Model file for the job. Use its own axes, mm. Face numbers are marked on the shaded views. A direction names the side the tool comes from. Round coordinates to 2 decimals unless told otherwise and drop trailing zeros. Order: outer loops, then holes, each group sorted by start corner. A loop starts at its lowest first (then second) coordinate and runs counter-clockwise, first axis right, second up. Notation, with made-up numbers: M -30,-32 L 15,-32 A23 cw 15,-12 Z; hole C 54.25,-31 d4. An arc over 180 degrees is marked long. Return JSON: item names as keys, results as strings. Group by question number.
Item 1: Pin check, flat tips, straight feed: pin 1 Ø13 at (x, z) = (8, -2.5) entering from -Y; pin 2 Ø5 at (x, z) = (-2, -0.5) entering from +Y. Stop position of each tip, or through.
Item 2: Probe line 1 along Z through (x, y) = (0, -2); line 2 along Z through (x, y) = (-1.5, -6.5); line 3 along X through (y, z) = (-6.25, 5.75). List the from-to ranges inside material, lowest first.
Item 3: Pull direction X, two halves, no side cores. Call the marked faces 3, 4 and 5: pulls with the +X half, pulls with the -X half, needs draft (parallel to the pull), parting line crosses it, or undercut.
Item 4: Slice it at A-A on z = 0. Write the cut outline in (x, y), then the cut area to 3 significant figures.
Item 5: Which spindle directions (+Z, -Z, +X, -X, +Y, -Y) get a long thin tool onto all of the face, cutting with end or side? Do the marked faces 1 and 2. Say none if no direction does.
Item 6: Slice it at B-B on x = -14.5. Write the cut outline in (y, z), then the cut area to 3 significant figures.
Item 7: Slice it at D-D on z = -9.75. Write the cut outline in (x, y).
Item 8: Slice it at C-C on y = -1.5. Write the cut outline in (x, z), then the cut area to 3 significant figures.
from build123d import *

# Parameters (mm, degrees)
F0_W     = 50
F0_H     = 30
F0_W_2   = 46
F0_H_2   = 26
F0_R     = 8
F0_R_2   = 5
F1_DEPTH = 5
F2_DEPTH = 7
F3_DEPTH = 3.0000000261


with BuildPart() as f1:
    # F0 (on Front) → F1 (new body)
    with BuildSketch(Plane.XZ):
        Rectangle(F0_W, F0_H)
        Rectangle(F0_W_2, F0_H_2, mode=Mode.SUBTRACT)
        Rectangle(F0_W_2, F0_H_2)
        Circle(F0_R, mode=Mode.SUBTRACT)
        Circle(F0_R)
        Circle(F0_R_2, mode=Mode.SUBTRACT)
        Circle(F0_R_2)
    extrude(amount=F1_DEPTH)

    # F0 (on Front) → F2 (join)
    with BuildSketch(Plane.XZ):
        Rectangle(F0_W, F0_H)
        Rectangle(F0_W_2, F0_H_2, mode=Mode.SUBTRACT)
    extrude(amount=F2_DEPTH)

    # F0 (on Front) → F3 (cut)
    with BuildSketch(Plane.XZ):
        Circle(F0_R_2)
    extrude(amount=F3_DEPTH, mode=Mode.SUBTRACT)


solid = f1.part
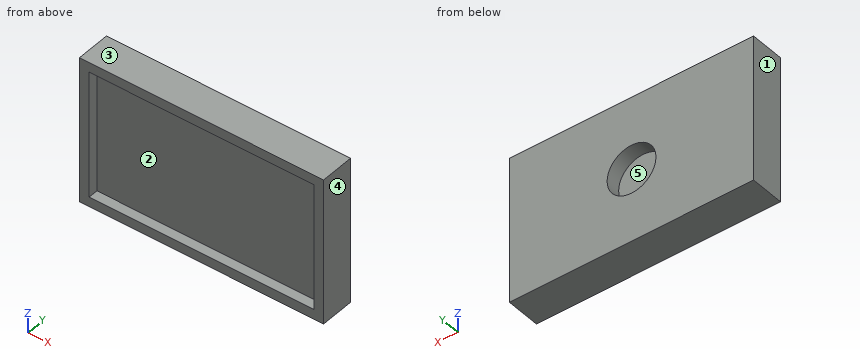
Output values:
{
 "1": {"pin 1": "y = -5", "pin 2": "y = -3"},
 "2": {"line 1": "-15 to -5, 5 to 15", "line 2": "-15 to -13, 13 to 15", "line 3": "-25 to -23, 23 to 25"},
 "3": {"face 3": "needs draft", "face 4": "pulls with the +X half", "face 5": "undercut"},
 "4": {"outline": "M -25,-7 L -23,-7 L -23,-5 L 23,-5 L 23,-7 L 25,-7 L 25,0 L 5,0 L 5,-3 L -5,-3 L -5,0 L -25,0 Z", "area": "228 mm²"},
 "5": {"face 1": "+Z, -Z, -X, +Y, -Y", "face 2": "-Y"},
 "6": {"outline": "M -7,-15 L 0,-15 L 0,15 L -7,15 L -7,13 L -5,13 L -5,-13 L -7,-13 Z", "area": "158 mm²"},
 "7": {"outline": "M -25,-7 L -23,-7 L -23,-5 L 23,-5 L 23,-7 L 25,-7 L 25,0 L -25,0 Z"},
 "8": {"outline": "M -25,-15 L 25,-15 L 25,15 L -25,15 Z; hole C 0,0 d10", "area": "1,420 mm²"}
}
